```python
from build123d import *

# Parameters (mm, degrees)
SKETCH1_R           = 5.1435
BOSS_EXTRUDE1_DEPTH = 10.3
BOSS_EXTRUDE2_DEPTH = 7.5
SKETCH3_R           = 10.75
BOSS_EXTRUDE3_DEPTH = 30.48
SKETCH4_R           = 9.525
BOSS_EXTRUDE4_DEPTH = 1.5
SKETCH5_R           = 8.255
BOSS_EXTRUDE5_DEPTH = 12
SKETCH6_R           = 10
BOSS_EXTRUDE6_DEPTH = 11.4
SKETCH7_R           = 4.3053
CUT_EXTRUDE1_DEPTH  = 11.4
SKETCH28_R          = 4.3053
BOSS_EXTRUDE7_DEPTH = 11.4
SKETCH29_R          = 1.5
CUT_EXTRUDE2_DEPTH  = 11.4
SKETCH30_R          = 9.525
CUT_EXTRUDE6_DEPTH  = 10.638
SKETCH31_W          = 0.381
SKETCH31_H          = 3.44369911
SKETCH31_W_2        = 3.44369911
SKETCH31_H_2        = 0.381
BOSS_EXTRUDE8_DEPTH = 7.239
CUT_EXTRUDE7_DEPTH  = 6.731
CUT_EXTRUDE8_DEPTH  = 1.651
CUT_EXTRUDE9_DEPTH  = 1.651
SKETCH35_R          = 9.525
BOSS_EXTRUDE9_DEPTH = 6.731


with BuildPart() as part:
    # Sketch1 → Boss-Extrude1 (new body)
    with BuildSketch(Plane(origin=(0, 0, 0), x_dir=(1, 0, 0), z_dir=(0, 1, 0))):
        Circle(SKETCH1_R)
    extrude(amount=BOSS_EXTRUDE1_DEPTH)

    # Sketch2 → Boss-Extrude2 (add)
    with BuildSketch(Plane(origin=(0, 10.3, 0), x_dir=(1, 0, 0), z_dir=(0, 1, 0))):
        Polygon((6.206515394, 10.75), (-6.206515394, 10.75), (-12.413030788, 0), (-6.206515394, -10.75), (6.206515394, -10.75), (12.413030788, 0), align=None)
    extrude(amount=BOSS_EXTRUDE2_DEPTH)

    # Sketch3 → Boss-Extrude3 (add)
    with BuildSketch(Plane(origin=(0, 17.8, 0), x_dir=(1, 0, 0), z_dir=(0, 1, 0))):
        Circle(SKETCH3_R)
    extrude(amount=BOSS_EXTRUDE3_DEPTH)

    # Sketch4 → Boss-Extrude4 (add)
    with BuildSketch(Plane(origin=(0, 48.28, 0), x_dir=(1, 0, 0), z_dir=(0, 1, 0))):
        Circle(SKETCH4_R)
    extrude(amount=BOSS_EXTRUDE4_DEPTH)

    # Sketch5 → Boss-Extrude5 (add)
    with BuildSketch(Plane(origin=(0, 49.78, 0), x_dir=(1, 0, 0), z_dir=(0, 1, 0))):
        Circle(SKETCH5_R)
    extrude(amount=BOSS_EXTRUDE5_DEPTH)

    # Sketch6 → Boss-Extrude6 (add)
    with BuildSketch(Plane(origin=(0, 61.78, 0), x_dir=(1, 0, 0), z_dir=(0, 1, 0))):
        Circle(SKETCH6_R)
    extrude(amount=BOSS_EXTRUDE6_DEPTH)

    # Sketch7 → Cut-Extrude1 (cut)
    with BuildSketch(Plane.XZ):
        Circle(SKETCH7_R)
    extrude(amount=-CUT_EXTRUDE1_DEPTH, mode=Mode.SUBTRACT)

    # Sketch28 → Boss-Extrude7 (add)
    with BuildSketch(Plane(origin=(0, 0, 0), x_dir=(-1, 0, 0), z_dir=(0, -1, 0))):
        Circle(SKETCH28_R)
    extrude(amount=-BOSS_EXTRUDE7_DEPTH)

    # Sketch29 → Cut-Extrude2 (cut)
    with BuildSketch(Plane.XZ):
        Circle(SKETCH29_R)
    extrude(amount=-CUT_EXTRUDE2_DEPTH, mode=Mode.SUBTRACT)

    # Sketch30 → Cut-Extrude6 (cut)
    with BuildSketch(Plane(origin=(0, 73.18, 0), x_dir=(1, 0, 0), z_dir=(0, 1, 0))):
        Circle(SKETCH30_R)
    extrude(amount=-CUT_EXTRUDE6_DEPTH, mode=Mode.SUBTRACT)

    # Sketch31 → Boss-Extrude8 (add)
    with BuildSketch(Plane(origin=(0, 62.542, 0), x_dir=(1, 0, 0), z_dir=(0, 1, 0))):
        with Locations((0, 3.0226)):
            Rectangle(SKETCH31_W, SKETCH31_H)
        with Locations((-2.2352, 0)):
            Rectangle(SKETCH31_W_2, SKETCH31_H_2)
        with Locations((2.2352, 0)):
            Rectangle(SKETCH31_W_2, SKETCH31_H_2)
    extrude(amount=BOSS_EXTRUDE8_DEPTH)

    # Sketch32 → Cut-Extrude7 (cut)
    with BuildSketch(Plane.XY.offset(0.1905)):
        Polygon((-3.957049555, 68.6888), (-2.2352, 69.781), (-3.957049555, 69.781), align=None)
        Polygon((-0.513350445, 69.781), (-2.2352, 69.781), (-0.513350445, 68.6888), align=None)
    extrude(amount=-CUT_EXTRUDE7_DEPTH, mode=Mode.SUBTRACT)

    # Sketch33 → Cut-Extrude8 (cut)
    with BuildSketch(Plane.XY.offset(0.1905)):
        Polygon((0.513350445, 68.6888), (2.2352, 69.781), (0.513350445, 69.781), align=None)
        Polygon((3.957049555, 69.781), (2.2352, 69.781), (3.957049555, 68.6888), align=None)
    extrude(amount=-CUT_EXTRUDE8_DEPTH, mode=Mode.SUBTRACT)

    # Sketch34 → Cut-Extrude9 (cut)
    with BuildSketch(Plane(origin=(0.1905, 0, 0), x_dir=(0, 0, -1), z_dir=(1, 0, 0))):
        Polygon((1.300750445, 68.6888), (3.0226, 69.781), (1.300750445, 69.781), align=None)
        Polygon((4.744449555, 69.781), (3.0226, 69.781), (4.744449555, 68.6888), align=None)
    extrude(amount=-CUT_EXTRUDE9_DEPTH, mode=Mode.SUBTRACT)

    # Sketch35 → Boss-Extrude9 (add)
    with BuildSketch(Plane(origin=(0, 62.542, 0), x_dir=(1, 0, 0), z_dir=(0, 1, 0))):
        Circle(SKETCH35_R)
        with BuildLine():
            ThreePointArc((-4.699, -3.683), (-0.167968835, -5.324730553), (4.363062329, -3.683))
            Line((4.363062329, -3.683), (4.363062329, -2.413))
            Line((4.363062329, -2.413), (5.715, -2.413))
            Line((5.715, -2.413), (5.715, 5.24229274))
            Line((5.715, 5.24229274), (3.860385896, 6.985))
            Line((3.860385896, 6.985), (-3.918948776, 6.985))
            Line((-3.918948776, 6.985), (-5.715, 5.188948776))
            Line((-5.715, 5.188948776), (-5.715, -2.413))
            Line((-5.715, -2.413), (-4.699, -2.413))
            Line((-4.699, -2.413), (-4.699, -3.683))
        make_face(mode=Mode.SUBTRACT)
    extrude(amount=BOSS_EXTRUDE9_DEPTH)


solid = part.part
```
Part model, mm, in its own coordinate system. A direction names the side the tool comes from. Give positions to 0.01 mm unless a question says otherwise; leave off trailing zeros. Write each loop counter-clockwise with the first axis right and the second up, starting at its lowest first coordinate (ties: lowest second). Pieces come first, ordered by that corner, then holes. Notation, with made-up numbers: (12.5, 14) -> (64.5, 14) arc R30 ccw to (64.5, 41) -> close; hole circle Ø7 at (81.25, -7.75). An arc over 180 degrees is marked (long way). Put each result on its own line as item: value. Start each with the question number.
Item 1: Pull direction Y, two halves, no side cores. Call faces 1 (the face through (-7.559, 49.02, 5.796)), 2 (the face through (-1, 48.28, 10)), 3 (the face through (4.8, 65.9, -6.1)), 4 (the face through (4.1, 69.273, 4.1)): pulls with the +Y half, pulls with the -Y half, needs draft (parallel to the pull), parting line crosses it, or undercut.
Item 2: Which spindle directions (+Z, -Z, +X, -X, +Y, -Y) get a long thin tool onto all of the face, cutting with end or side? Do faces 5 (the face through (11, 17.8, 0)), 6 (the face through (6, 17.8, 10)), 7 (the face through (-0.19, 66, -3)). Say none if no direction does.
Item 3: Wall check: L1, parallel to X at y = 64.5, z = 0 (3 decimals); L2, parallel to Z at x = 0, y = 4; L3, parallel to X at y = 71.05, z = 0 (3 decimals). Give the ranges that are in metal, low to high. Write a range as [from, to].
Item 4: Cut at B-B (y = 53.5). List the corners of the cut face in (x, z) (3 decimals), then the cut area to 3 significant figures.
Item 5: Cut at C-C (y = 29.5). List the corners of the cut face in (x, z), then the cut area to 3 significant figures.
Item 6: Pin check, flat tips, straight feed: pin 1 Ø3 at (x, y) = (-1.5, 67.5) entering from -Z; pin 2 Ø9.5 at (x, z) = (2, 1.5) entering from +Y; pin 3 Ø3.5 at (x, y) = (1.5, 64.5) entering from +Z. Stop position of each tip, or through.
Answer list:
1. face 1: undercut
1. face 2: undercut
1. face 3: needs draft
1. face 4: pulls with the +Y half
2. face 5: +X, +Y
2. face 6: +Z, +X, +Y
2. face 7: +Y
3. L1: x = [-10, -5.715], [-3.957, -0.513], [0.513, 3.957], [5.715, 10]
3. L2: z = [-5.14, -1.5], [1.5, 5.14]
3. L3: x = [-10, -9.525], [9.525, 10]
4. outline: circle Ø16.51 at (0, 0)
4. area: 214 mm2
5. outline: circle Ø21.5 at (0, 0)
5. area: 363 mm2
6. pin 1: stops at z = -10
6. pin 2: stops at y = 69.78
6. pin 3: stops at z = 10
